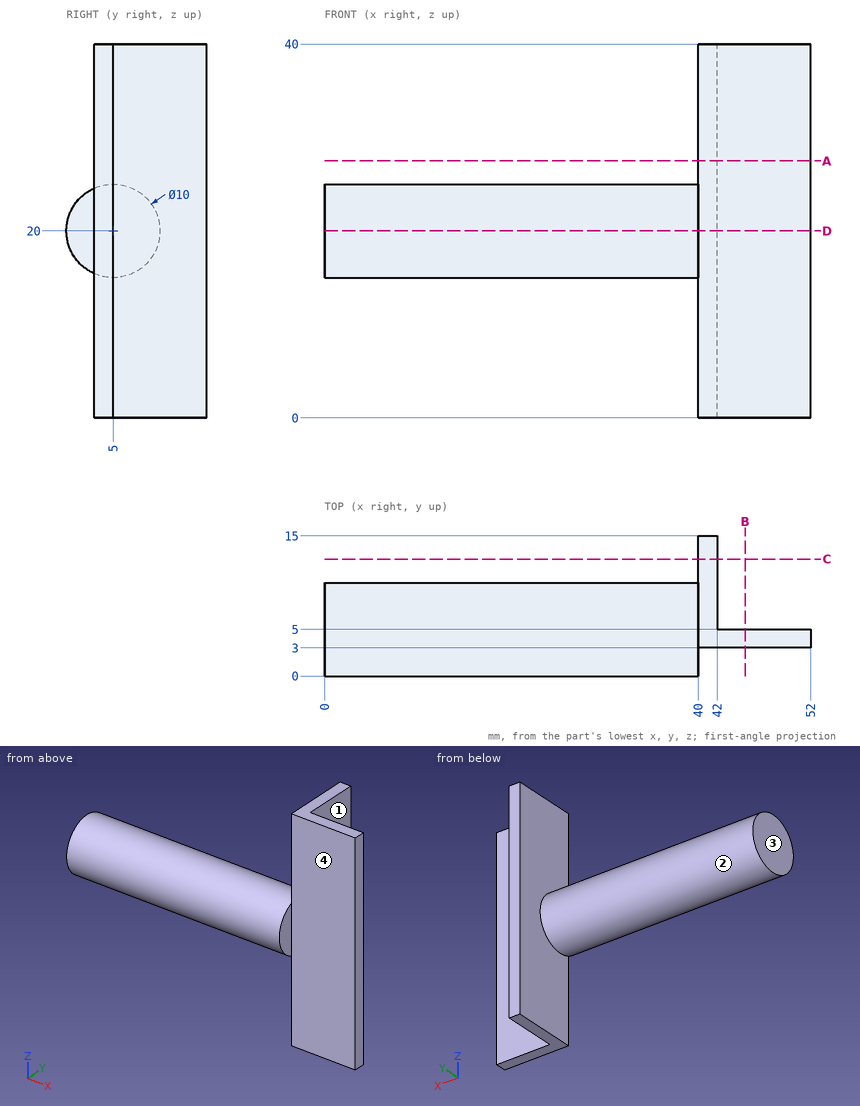
The drawing under review shows one solid part. Ordinate dimensions are in mm from its lowest x, y, z. A direction names the side the tool comes from. Coordinates: 2 decimals unless noted, no trailing zeros. Order: outer loops, then holes, each group sorted by start corner. A loop starts at its lowest first (then second) coordinate and runs counter-clockwise, first axis right, second up. Notation, with made-up numbers: (-20.5, 79.25) -> (38.5, 79.25) arc R30 ccw to (38.5, 111.25) -> close; hole circle Ø10 at (-19.5, -18). An arc over 180 degrees is marked (long way). Answer in a Markdown table with one row per item. Add a question column.
Item 1: We need section C-C on y = 12.5. Write out the cut boundary in (x, z).
Item 2: We need section B-B on x = 45. Write out the cut boundary in (y, z).
Item 3: To check wall thickness, follow probe 1 along X at (y, z) = (9, 10.5); probe 2 along X at (y, z) = (3.5, 27); probe 3 along Y at (x, z) = (46, 18). State the ranges of each line that lie inside material, in increasing order.
Item 4: We need section A-A on z = 27.5. Write out the cut boundary in (x, y).
Item 5: Machinability: for the marked faces 1, 2, 3 and 4, which of the approach directions +Z, -Z, +X, -X, +Y, -Y give a long, thin tool a straight path to every point of the face, cutting with its end or side? Answer none if there is none.
Item 6: Clearance check with flat-ended pins moving along their axes: pin 1 (9.5 mm diameter, centred on x = 45.5, z = 29, fed in from -Y); pin 2 (3 mm diameter, centred on x = 20.5, y = 6, fed in from -Z); pin 3 (11 mm diameter, centred on x = 47, z = 22, fed in from +Y); pin 4 (8 mm diameter, centred on y = 9.5, z = 18, fed in from +X). State where each tip first meets the part, or that it passes through.
Item 7: We need section D-D on z = 20. Write out the cut boundary in (x, y), plus the area to 3 significant figures.
Final values:
| question | item | result |
|---|---|---|
| 1 | outline | (40, 0) -> (42, 0) -> (42, 40) -> (40, 40) -> close |
| 2 | outline | (3, 0) -> (5, 0) -> (5, 40) -> (3, 40) -> close |
| 3 | probe 1 | x = 40 to 42 |
| 3 | probe 2 | x = 40 to 52 |
| 3 | probe 3 | y = 3 to 5 |
| 4 | outline | (40, 3) -> (52, 3) -> (52, 5) -> (42, 5) -> (42, 15) -> (40, 15) -> close |
| 5 | face 1 | +Z, -Z, +X, +Y |
| 5 | face 2 | -X |
| 5 | face 3 | +Z, -Z, -X, +Y, -Y |
| 5 | face 4 | +Z, -Z, +X, -Y |
| 6 | pin 1 | stops at y = 3 |
| 6 | pin 2 | stops at z = 15 |
| 6 | pin 3 | stops at y = 15 |
| 6 | pin 4 | stops at x = 42 |
| 7 | outline | (0, 0) -> (40, 0) -> (40, 3) -> (52, 3) -> (52, 5) -> (42, 5) -> (42, 15) -> (40, 15) -> (40, 10) -> (0, 10) -> close |
| 7 | area | 444 mm2 |
